Work out the finished part from the listing and answer in its coordinate system (mm). Face numbers are marked on the shaded views. A direction names the side the tool comes from. Coordinates: 2 decimals unless noted, no trailing zeros. Order: outer loops, then holes, each group sorted by start corner. A loop starts at its lowest first (then second) coordinate and runs counter-clockwise, first axis right, second up.
1. Find the intervals of material crossed by probe 1 along X at (y, z) = (-45.5, 23); probe 2 along Z at (x, y) = (-9.75, 0); probe 3 along X at (y, z) = (-3, -20), in increasing order.
2. The part is cut by section B-B, the plane x = 34. Give the vertices of the cut face in (y, z), then the cut area to 3 significant figures.
3. A tool of negligible diameter and unlimited length cuts with its end or side. For the marked faces 1 and 2, from which of +Z, -Z, +X, -X, +Y, -Y can it reach the whole face along a straight path? Write none if from no direction.
4. The part is cut by section A-A, the plane x = -4. Give the vertices of the cut face in (y, z) (1 decimal).
5. Determine the mould class of the marked faces 3, 4 and 5 for opening direction X: +X half, -X half, draft (parallel to the pull), parting line (faces both ways), or undercut.
6. Flat-ended cylindrical pins translate along their axes: pin 1 Ø4 at (x, y) = (0, 14) entering from +Z; pin 2 Ø2.5 at (y, z) = (52.8, -21.87) entering from -X; pin 3 Ø5 at (x, z) = (44.5, -22.5) entering from -Y. Find the tip coordinate at first contact, or state that the pin passes through.
```python
from build123d import *

# Parameters (mm, degrees)
SKETCH2_R          = 50.00625
SKETCH2_R_2        = 47.625
CUT_EXTRUDE1_DEPTH = 1.190625
CUT_EXTRUDE2_REACH = 118.086
SKETCH3_R          = 1.5875


with BuildPart() as part:
    # Sketch1 → Revolve1 (revolve)
    with BuildSketch(Plane.XY):
        Polygon((0, 15.5575), (83.038845842, 63.5), (83.038845842, 57.15), (0, 7.9375), (-12.7, 7.9375), (-33.047266862, 41.275), (-33.047266862, 50.8), (-33.047266862, 63.5), (-20.347266862, 63.5), (-20.347266862, 28.802954744), (-12.7, 15.5575), align=None)
    revolve(axis=Axis((0, 0, 0), (1, 0, 0)))

    # Sketch2 → Cut-Extrude1 (cut)
    with BuildSketch(Plane.ZY.offset(33.047266862)):
        Circle(SKETCH2_R)
        Circle(SKETCH2_R_2, mode=Mode.SUBTRACT)
    extrude(amount=-CUT_EXTRUDE1_DEPTH, mode=Mode.SUBTRACT)

    # Sketch3 → Cut-Extrude2 (cut, up to next)
    with BuildSketch(Plane.ZY.offset(33.047266862), mode=Mode.PRIVATE) as cut_extrude2_sk1:
        with Locations((0, 57.15)):
            Circle(SKETCH3_R)
    cut_extrude2_tool1 = extrude(cut_extrude2_sk1.sketch, amount=-CUT_EXTRUDE2_REACH, mode=Mode.PRIVATE) & part.part
    add(cut_extrude2_tool1.solids().sort_by_distance((-33.047267, 57.15, 0))[0], mode=Mode.SUBTRACT)
    # Sketch3 → Cut-Extrude2 (cut, up to next)
    with BuildSketch(Plane.ZY.offset(33.047266862), mode=Mode.PRIVATE) as cut_extrude2_sk2:
        with Locations((21.87035816, 52.799715283)):
            Circle(SKETCH3_R)
    cut_extrude2_tool2 = extrude(cut_extrude2_sk2.sketch, amount=-CUT_EXTRUDE2_REACH, mode=Mode.PRIVATE) & part.part
    add(cut_extrude2_tool2.solids().sort_by_distance((-33.047267, 52.799715, 21.870358))[0], mode=Mode.SUBTRACT)
    # Sketch3 → Cut-Extrude2 (cut, up to next)
    with BuildSketch(Plane.ZY.offset(33.047266862), mode=Mode.PRIVATE) as cut_extrude2_sk3:
        with Locations((40.411152545, 40.411152545)):
            Circle(SKETCH3_R)
    cut_extrude2_tool3 = extrude(cut_extrude2_sk3.sketch, amount=-CUT_EXTRUDE2_REACH, mode=Mode.PRIVATE) & part.part
    add(cut_extrude2_tool3.solids().sort_by_distance((-33.047267, 40.411153, 40.411153))[0], mode=Mode.SUBTRACT)
    # Sketch3 → Cut-Extrude2 (cut, up to next)
    with BuildSketch(Plane.ZY.offset(33.047266862), mode=Mode.PRIVATE) as cut_extrude2_sk4:
        with Locations((52.799715283, 21.87035816)):
            Circle(SKETCH3_R)
    cut_extrude2_tool4 = extrude(cut_extrude2_sk4.sketch, amount=-CUT_EXTRUDE2_REACH, mode=Mode.PRIVATE) & part.part
    add(cut_extrude2_tool4.solids().sort_by_distance((-33.047267, 21.870358, 52.799715))[0], mode=Mode.SUBTRACT)
    # Sketch3 → Cut-Extrude2 (cut, up to next)
    with BuildSketch(Plane.ZY.offset(33.047266862), mode=Mode.PRIVATE) as cut_extrude2_sk5:
        with Locations((57.15, 0)):
            Circle(SKETCH3_R)
    cut_extrude2_tool5 = extrude(cut_extrude2_sk5.sketch, amount=-CUT_EXTRUDE2_REACH, mode=Mode.PRIVATE) & part.part
    add(cut_extrude2_tool5.solids().sort_by_distance((-33.047267, 0, 57.15))[0], mode=Mode.SUBTRACT)
    # Sketch3 → Cut-Extrude2 (cut, up to next)
    with BuildSketch(Plane.ZY.offset(33.047266862), mode=Mode.PRIVATE) as cut_extrude2_sk6:
        with Locations((52.799715283, -21.87035816)):
            Circle(SKETCH3_R)
    cut_extrude2_tool6 = extrude(cut_extrude2_sk6.sketch, amount=-CUT_EXTRUDE2_REACH, mode=Mode.PRIVATE) & part.part
    add(cut_extrude2_tool6.solids().sort_by_distance((-33.047267, -21.870358, 52.799715))[0], mode=Mode.SUBTRACT)
    # Sketch3 → Cut-Extrude2 (cut, up to next)
    with BuildSketch(Plane.ZY.offset(33.047266862), mode=Mode.PRIVATE) as cut_extrude2_sk7:
        with Locations((40.411152545, -40.411152545)):
            Circle(SKETCH3_R)
    cut_extrude2_tool7 = extrude(cut_extrude2_sk7.sketch, amount=-CUT_EXTRUDE2_REACH, mode=Mode.PRIVATE) & part.part
    add(cut_extrude2_tool7.solids().sort_by_distance((-33.047267, -40.411153, 40.411153))[0], mode=Mode.SUBTRACT)
    # Sketch3 → Cut-Extrude2 (cut, up to next)
    with BuildSketch(Plane.ZY.offset(33.047266862), mode=Mode.PRIVATE) as cut_extrude2_sk8:
        with Locations((21.87035816, -52.799715283)):
            Circle(SKETCH3_R)
    cut_extrude2_tool8 = extrude(cut_extrude2_sk8.sketch, amount=-CUT_EXTRUDE2_REACH, mode=Mode.PRIVATE) & part.part
    add(cut_extrude2_tool8.solids().sort_by_distance((-33.047267, -52.799715, 21.870358))[0], mode=Mode.SUBTRACT)
    # Sketch3 → Cut-Extrude2 (cut, up to next)
    with BuildSketch(Plane.ZY.offset(33.047266862), mode=Mode.PRIVATE) as cut_extrude2_sk9:
        with Locations((0, -57.15)):
            Circle(SKETCH3_R)
    cut_extrude2_tool9 = extrude(cut_extrude2_sk9.sketch, amount=-CUT_EXTRUDE2_REACH, mode=Mode.PRIVATE) & part.part
    add(cut_extrude2_tool9.solids().sort_by_distance((-33.047267, -57.15, 0))[0], mode=Mode.SUBTRACT)
    # Sketch3 → Cut-Extrude2 (cut, up to next)
    with BuildSketch(Plane.ZY.offset(33.047266862), mode=Mode.PRIVATE) as cut_extrude2_sk10:
        with Locations((-21.87035816, -52.799715283)):
            Circle(SKETCH3_R)
    cut_extrude2_tool10 = extrude(cut_extrude2_sk10.sketch, amount=-CUT_EXTRUDE2_REACH, mode=Mode.PRIVATE) & part.part
    add(cut_extrude2_tool10.solids().sort_by_distance((-33.047267, -52.799715, -21.870358))[0], mode=Mode.SUBTRACT)
    # Sketch3 → Cut-Extrude2 (cut, up to next)
    with BuildSketch(Plane.ZY.offset(33.047266862), mode=Mode.PRIVATE) as cut_extrude2_sk11:
        with Locations((-40.411152545, -40.411152545)):
            Circle(SKETCH3_R)
    cut_extrude2_tool11 = extrude(cut_extrude2_sk11.sketch, amount=-CUT_EXTRUDE2_REACH, mode=Mode.PRIVATE) & part.part
    add(cut_extrude2_tool11.solids().sort_by_distance((-33.047267, -40.411153, -40.411153))[0], mode=Mode.SUBTRACT)
    # Sketch3 → Cut-Extrude2 (cut, up to next)
    with BuildSketch(Plane.ZY.offset(33.047266862), mode=Mode.PRIVATE) as cut_extrude2_sk12:
        with Locations((-52.799715283, -21.87035816)):
            Circle(SKETCH3_R)
    cut_extrude2_tool12 = extrude(cut_extrude2_sk12.sketch, amount=-CUT_EXTRUDE2_REACH, mode=Mode.PRIVATE) & part.part
    add(cut_extrude2_tool12.solids().sort_by_distance((-33.047267, -21.870358, -52.799715))[0], mode=Mode.SUBTRACT)
    # Sketch3 → Cut-Extrude2 (cut, up to next)
    with BuildSketch(Plane.ZY.offset(33.047266862), mode=Mode.PRIVATE) as cut_extrude2_sk13:
        with Locations((-57.15, 0)):
            Circle(SKETCH3_R)
    cut_extrude2_tool13 = extrude(cut_extrude2_sk13.sketch, amount=-CUT_EXTRUDE2_REACH, mode=Mode.PRIVATE) & part.part
    add(cut_extrude2_tool13.solids().sort_by_distance((-33.047267, 0, -57.15))[0], mode=Mode.SUBTRACT)
    # Sketch3 → Cut-Extrude2 (cut, up to next)
    with BuildSketch(Plane.ZY.offset(33.047266862), mode=Mode.PRIVATE) as cut_extrude2_sk14:
        with Locations((-52.799715283, 21.87035816)):
            Circle(SKETCH3_R)
    cut_extrude2_tool14 = extrude(cut_extrude2_sk14.sketch, amount=-CUT_EXTRUDE2_REACH, mode=Mode.PRIVATE) & part.part
    add(cut_extrude2_tool14.solids().sort_by_distance((-33.047267, 21.870358, -52.799715))[0], mode=Mode.SUBTRACT)
    # Sketch3 → Cut-Extrude2 (cut, up to next)
    with BuildSketch(Plane.ZY.offset(33.047266862), mode=Mode.PRIVATE) as cut_extrude2_sk15:
        with Locations((-40.411152545, 40.411152545)):
            Circle(SKETCH3_R)
    cut_extrude2_tool15 = extrude(cut_extrude2_sk15.sketch, amount=-CUT_EXTRUDE2_REACH, mode=Mode.PRIVATE) & part.part
    add(cut_extrude2_tool15.solids().sort_by_distance((-33.047267, 40.411153, -40.411153))[0], mode=Mode.SUBTRACT)
    # Sketch3 → Cut-Extrude2 (cut, up to next)
    with BuildSketch(Plane.ZY.offset(33.047266862), mode=Mode.PRIVATE) as cut_extrude2_sk16:
        with Locations((-21.87035816, 52.799715283)):
            Circle(SKETCH3_R)
    cut_extrude2_tool16 = extrude(cut_extrude2_sk16.sketch, amount=-CUT_EXTRUDE2_REACH, mode=Mode.PRIVATE) & part.part
    add(cut_extrude2_tool16.solids().sort_by_distance((-33.047267, 52.799715, -21.870358))[0], mode=Mode.SUBTRACT)


solid = part.part
```
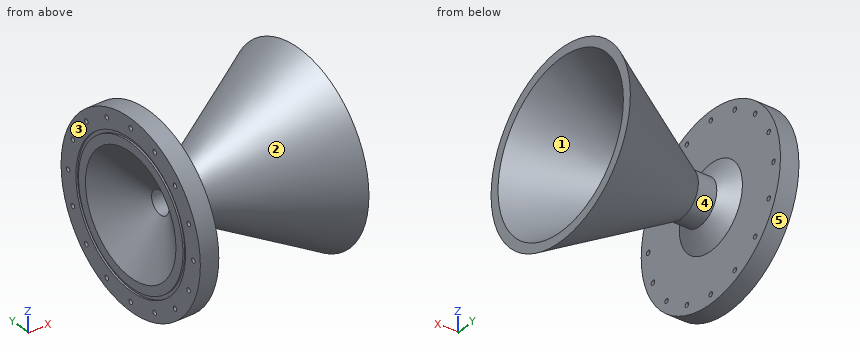
Geometry says:
1. probe 1: x = -33.05 to -20.35, 61.36 to 72.63
1. probe 2: z = -15.56 to -7.94, 7.94 to 15.56
1. probe 3: x = -20.2 to -15.39, 8.08 to 20.73
2. outline: circle Ø70.37 at (0, 0); hole circle Ø56.17 at (0, 0)
2. area: 1,410 mm2
3. face 1: +X
3. face 2: none
4. outline: circle Ø31.1 at (0, 0); hole circle Ø15.9 at (0, 0)
5. face 3: -X half
5. face 4: undercut
5. face 5: draft
6. pin 1: stops at z = 10.5
6. pin 2: stops at x = 69.88
6. pin 3: stops at y = -36.84
